Source: CAD feature listing. Evaluate the final solid. Frame: model axes, mm. A direction names the side the tool comes from. Give positions to 0.01 mm unless a question says otherwise; leave off trailing zeros. Loops run counter-clockwise (first coordinate to the right, second up) from the corner with the lowest first, then second, coordinate; pieces in that order, holes last. Notation, with made-up numbers: M 24.5,7 L 60.5,7 A30 ccw 60.5,29 Z; hole C 49.25,-4 d9. An arc over 180 degrees is marked long. Write item = value, one per line.
from build123d import *

# Parameters (mm, degrees)
SKIZZE1_W                       = 4
SKIZZE1_H                       = 20
SKIZZE5_W                       = 10
SKIZZE5_H                       = 10
AUFSATZ_LINEAR_AUSTRAGEN1_DEPTH = 10
M5_GEWINDEBOHRUNG2_D            = 4.2


with BuildPart() as part:
    # Skizze1 → Rotation1 (revolve)
    with BuildSketch(Plane.XY, mode=Mode.PRIVATE) as rotation1_sk:
        with Locations((2, 10)):
            Rectangle(SKIZZE1_W, SKIZZE1_H)
    revolve(rotation1_sk.sketch.rotate(Axis((0, -2.459302686, 0), (0, 1, 0)), 90), axis=Axis((0, -2.459302686, 0), (0, 1, 0)))

    # Skizze5 → Aufsatz-Linear austragen1 (add)
    with BuildSketch(Plane(origin=(0, 20, 0), x_dir=(1, 0, 0), z_dir=(0, 1, 0))):
        Rectangle(SKIZZE5_W, SKIZZE5_H)
    extrude(amount=AUFSATZ_LINEAR_AUSTRAGEN1_DEPTH)

    # M5 Gewindebohrung2 (through all)
    with Locations(Plane(origin=(0, 30, 0), x_dir=(1, 0, 0), z_dir=(0, 1, 0))):
        with Locations((0, 0)):
            Hole(M5_GEWINDEBOHRUNG2_D / 2)


solid = part.part
1. Cut plane C-C, the plane y = 25.5. Return the cut outline in (x, z), then the cut area to 3 significant figures.
Derived:
outline = M -5,-5 L 5,-5 L 5,5 L -5,5 Z; hole C 0,0 d4.2
area = 86.1 mm²
2. Cut plane B-B, the plane z = 0. Return the cut outline in (x, y), then the cut area to 3 significant figures.
Derived:
outline = M -5,20 L -4,20 L -4,0 L -2.1,0 L -2.1,30 L -5,30 Z; M 2.1,0 L 4,0 L 4,20 L 5,20 L 5,30 L 2.1,30 Z
area = 134 mm²
3. Material intervals for probe 1 along Y at (x, z) = (4.25, -2); probe 2 along X at (y, z) = (20.25, -1.75); probe 3 along Z at (x, y) = (-0.5, 18.5), sorted ascending. Write a range as from..to.
Derived:
probe_1 = 20..30
probe_2 = -5..-1.16, 1.16..5
probe_3 = -3.97..-2.04, 2.04..3.97
4. Cut plane A-A, the plane x = 0. Return the cut outline in (y, z).
Derived:
outline = M 0,-4 L 20,-4 L 20,-5 L 30,-5 L 30,-2.1 L 0,-2.1 Z; M 0,2.1 L 30,2.1 L 30,5 L 20,5 L 20,4 L 0,4 Z
5. Cut plane D-D, the plane x = -3.5. Return the cut outline in (y, z).
Derived:
outline = M 0,-1.94 L 20,-1.94 L 20,-5 L 30,-5 L 30,5 L 20,5 L 20,1.94 L 0,1.94 Z
6. Pull-direction query (Z, two-part tool) for faces 1 (the flat face through (2, 0, 2)), 2 (the cylindrical face through (-2.003, 14.79, -0.631)), 3 (the cylindrical face through (3.905, 10.14, 0.867)), 4 (the flat face through (0, 25, 5)); classes: +Z half, -Z half, draft (parallel to the pull), parting line (faces both ways), or undercut.
Derived:
face_1 = draft
face_2 = undercut
face_3 = parting line
face_4 = +Z half
7. Reachability of faces 5 (the flat face through (0, 25, -5)), 6 (the flat face through (-4.5, 20, -0.1)) from +Z, -Z, +X, -X, +Y, -Y: full face, straight path, thin tool, end or side. Return the list, or none.
Derived:
face_5 = -Z, +X, -X, +Y, -Y
face_6 = -Y
8. First-contact query: pin 1 Ø1.5 at (y, z) = (13.5, -1.5) entering from -X; pin 2 Ø1 at (x, y) = (3.5, 15) entering from -Z; pin 3 Ø1.5 at (x, z) = (-1.5, 1.5) entering from -Y; pin 4 Ø1.5 at (x, z) = (4, -3) entering from -Y. Flat tips, straight axial feed; report the tip coordinate or a pass-through.
Derived:
pin_1 = -3.93
pin_2 = -2.65
pin_3 = 0
pin_4 = 20
